Work out the finished part from the listing and answer in its coordinate system (mm). Face numbers are marked on the shaded views. A direction names the side the tool comes from. Coordinates: 2 decimals unless noted, no trailing zeros. Order: outer loops, then holes, each group sorted by start corner. A loop starts at its lowest first (then second) coordinate and runs counter-clockwise, first axis right, second up.
1. Determine the mould class of the marked faces 3, 4, 5 and 6 for opening direction Y: +Y half, -Y half, draft (parallel to the pull), parting line (faces both ways), or undercut.
2. Find the intervals of material crossed by probe 1 along X at (y, z) = (-63, 2.75); probe 2 along Z at (x, y) = (-4.75, -61.5); probe 3 along Y at (x, z) = (-8, 4.5), in increasing order.
3. A tool of negligible diameter and unlimited length cuts with its end or side. For the marked faces 1 and 2, from which of +Z, -Z, +X, -X, +Y, -Y can it reach the whole face along a straight path? Write none if from no direction.
4. Flat-ended cylindrical pins translate along their axes: pin 1 Ø1 at (y, z) = (-66.5, 2.5) entering from +X; pin 2 Ø2 at (y, z) = (-34, 2) entering from -X; pin 3 Ø12 at (x, y) = (5.5, -48.5) entering from +Z. Find the tip coordinate at first contact, or state that the pin passes through.
5. The part is cut by section A-A, the plane x = 0. Give the vertices of the cut face in (y, z), then the cut area to 3 significant figures.
6. The part is cut by section C-C, the plane x = 8. Give the vertices of the cut face in (y, z), then the cut area to 3 significant figures.
7. The part is cut by section B-B, the plane y = -30. Give the vertices of the cut face in (x, z).
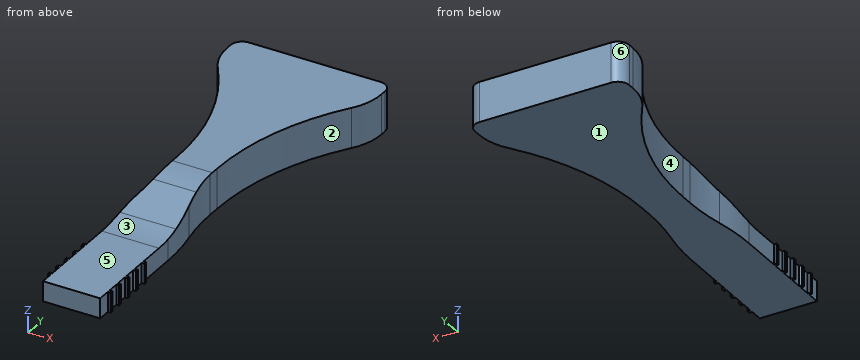
```python
from build123d import *

# Parameters (mm, degrees)
BOSS_EXTRUDE1_DEPTH     = 7
CUT_EXTRUDE4_DEPTH      = 72.7723837
CUT_EXTRUDE4_DEPTH_BACK = 72.7723837
FILLET2_R               = 20
SKETCH5_W               = 3.5
SKETCH5_H               = 0.5
BOSS_EXTRUDE2_DEPTH     = 0.5


with BuildPart() as part:
    # Sketch1 → Boss-Extrude1 (new body)
    with BuildSketch(Plane.XY):
        with BuildLine():
            Line((-5, -50.142890317), (-5, -70.142890317))
            Line((-5, -70.142890317), (5, -70.142890317))
            Line((5, -70.142890317), (5, -50.142890317))
            ThreePointArc((5, -50.142890317), (4.812033579, -46.374186959), (4.25, -42.642890317))
            ThreePointArc((4.25, -42.642890317), (3.687966421, -38.911593674), (3.5, -35.142890317))
            Line((3.5, -35.142890317), (3.5, -33.142890317))
            ThreePointArc((3.5, -33.142890317), (5.594183484, -19.574879811), (11.681818182, -7.269709461))
            ThreePointArc((11.681818182, -7.269709461), (13.034625892, -4.535227161), (13.5, -1.520113715))
            Line((13.5, -1.520113715), (13.5, -0.377223398))
            ThreePointArc((13.5, -0.377223398), (12.914213562, 1.036990164), (11.5, 1.622776602))
            Line((11.5, 1.622776602), (-11.5, 1.622776602))
            ThreePointArc((-11.5, 1.622776602), (-12.914213562, 1.036990164), (-13.5, -0.377223398))
            Line((-13.5, -0.377223398), (-13.5, -1.520113715))
            ThreePointArc((-13.5, -1.520113715), (-13.034625892, -4.535227161), (-11.681818182, -7.269709461))
            ThreePointArc((-11.681818182, -7.269709461), (-5.594183484, -19.574879811), (-3.5, -33.142890317))
            Line((-3.5, -33.142890317), (-3.5, -35.142890317))
            ThreePointArc((-3.5, -35.142890317), (-3.687966421, -38.911593674), (-4.25, -42.642890317))
            ThreePointArc((-4.25, -42.642890317), (-4.812033579, -46.374186959), (-5, -50.142890317))
        make_face()
    extrude(amount=BOSS_EXTRUDE1_DEPTH)

    # Sketch4 → Cut-Extrude4 (cut, two sides: drawn at the far end of the back side and taken through both)
    with BuildSketch(Plane(origin=(0, 0, 0), x_dir=(0, 0, -1), z_dir=(1, 0, 0)).offset(-CUT_EXTRUDE4_DEPTH_BACK)):
        Polygon((-3.5, -70.142890317), (-3.5, -50.142890317), (-7, -37.142890317), (-7, -70.142890317), align=None)
    extrude(amount=CUT_EXTRUDE4_DEPTH + CUT_EXTRUDE4_DEPTH_BACK, mode=Mode.SUBTRACT)

    # Fillet2
    fillet2_edges = [part.edges().sort_by_distance(p)[0] for p in [
        (0, -37.142890317, 7),
        (0, -50.142890317, 3.5),
    ]]
    fillet(fillet2_edges, radius=FILLET2_R)

    # Sketch5 → Boss-Extrude2 (add)
    with BuildSketch(Plane.ZY.offset(5)):
        with Locations((1.75, -65.142890317)):
            Rectangle(SKETCH5_W, SKETCH5_H)
        with Locations((1.75, -62.642890317)):
            Rectangle(SKETCH5_W, SKETCH5_H)
        with Locations((1.75, -60.142890317)):
            Rectangle(SKETCH5_W, SKETCH5_H)
        with Locations((1.75, -67.642890317)):
            Rectangle(SKETCH5_W, SKETCH5_H)
        with Locations((1.75, -57.642890317)):
            Rectangle(SKETCH5_W, SKETCH5_H)
    boss_extrude2 = extrude(amount=BOSS_EXTRUDE2_DEPTH)

    # Mirror1: Boss-Extrude2 across plane
    add(boss_extrude2.mirror(Plane(origin=(0, 0, 0), x_dir=(0, 0, 1), z_dir=(1, 0, 0))))


solid = part.part
```
Geometry says:
1. face 3: -Y half
1. face 4: undercut
1. face 5: draft
1. face 6: +Y half
2. probe 1: x = -5 to 5
2. probe 2: z = 0 to 3.5
2. probe 3: y = -13.53 to 1.62
3. face 1: -Z, +X, -X, +Y, -Y
3. face 2: +Z, -Z, +X
4. pin 1: stops at x = 5
4. pin 2: stops at x = -3.5
4. pin 3: stops at z = 5.52
5. outline: (-70.14, 0) - (1.62, 0) - (1.62, 7) - (-34.5, 7) arc R20 ccw to (-39.7, 6.31) - (-47.59, 4.19) arc R20 cw to (-52.79, 3.5) - (-70.14, 3.5) - close
5. area: 410 mm2
6. outline: (-13.53, 0) - (1.62, 0) - (1.62, 7) - (-13.53, 7) - close
6. area: 106 mm2
7. outline: (-3.61, 0) - (3.61, 0) - (3.61, 7) - (-3.61, 7) - close
